Solid Edge part; units mm, degrees
sketch "Sketch1" plane through (0, 0, 0) normal (0, -1, 0) x (1, 0, 0)
  circle A0 centre (0, 0) radius 36.2077
extrude "Protrusion1" add sketch "Sketch1" against normal blind 6.35
extrude "Cutout1" [suppressed]
pattern "Pattern1" [suppressed]
hole "Hole_1" at (-22.225, 0, 0) direction (0, 1, 0) diameter 3.175 end up to next
hole "Hole1" at (22.225, 0, 0) direction (0, 1, 0) diameter 3.175 end up to next
Input: part model. Units: mm. Frame: model coordinates. Round coordinates to 2 decimals unless told otherwise and drop trailing zeros. Loops run counter-clockwise (first coordinate to the right, second up) from the corner with the lowest first, then second, coordinate; pieces in that order, holes last. Notation, with made-up numbers: M 54.5,70.5 L 79.5,70.5 A16 ccw 79.5,84.5 Z; hole C 52.5,37.5 d9. An arc over 180 degrees is marked long. Answer in a Markdown table with one row per item. Add a question column.
1. Contact query for flat-ended pins moving along their axis: pin 1 (3 mm diameter, centred on y = 5.5, z = -9.5, fed in from +X); pin 2 (1.5 mm diameter, centred on y = 1, z = -8.5, fed in from -X). Output: stop coordinate, or through.
2. Section C-C (x = -7). Output: boundary loops of the cut face in (y, z), and give its area (3 significant figures).
3. Section B-B (y = 1). Output: boundary loops of the cut face in (x, z) (1 decimal).
4. Mould query, pull axis Z, two halves, no side actions, for faces 1 (the face through (23.564, 3.131, -0.853)), 2 (the face through (1, 0, 1)), 3 (the face through (-28.733, 3.131, -22.032)), 4 (the face through (-20.65, 3.13, 0.21)). Classes: released by +Z, released by -Z, zero draft, split by the parting line, or undercut.
5. Section D-D (z = -27). Output: boundary loops of the cut face in (x, y), and give its area (3 significant figures).
6. Ray query, probe 1 along X at (y, z) = (3.5, 16); probe 2 along Z at (x, y) = (-26, 0.5); probe 3 along X at (y, z) = (5.25, -18). Return the intervals inside material, ascending.
7. Section A-A (z = 0). Output: boundary loops of the cut face in (x, y).
Values follow:
| question | item | result |
|---|---|---|
| 1 | pin 1 | x = 35.31 |
| 1 | pin 2 | x = -35.37 |
| 2 | outline | M 0,-35.52 L 6.35,-35.52 L 6.35,35.52 L 0,35.52 Z |
| 2 | area | 451 mm^2 |
| 3 | outline | C 0,0 d72.4; hole C -22.2,0 d3.2; hole C 22.2,0 d3.2 |
| 4 | face 1 | undercut |
| 4 | face 2 | zero draft |
| 4 | face 3 | split by the parting line |
| 4 | face 4 | undercut |
| 5 | outline | M -24.12,0 L 24.12,0 L 24.12,6.35 L -24.12,6.35 Z |
| 5 | area | 306 mm^2 |
| 6 | probe 1 | -32.48 to 32.48 |
| 6 | probe 2 | -25.2 to 25.2 |
| 6 | probe 3 | -31.42 to 31.42 |
| 7 | outline | M -36.21,0 L -23.81,0 L -23.81,6.35 L -36.21,6.35 Z; M -20.64,0 L 20.64,0 L 20.64,6.35 L -20.64,6.35 Z; M 23.81,0 L 36.21,0 L 36.21,6.35 L 23.81,6.35 Z |
